Part print with two shaded views. Sizes in mm from the minimum x, y, z corner. Give positions to 0.01 mm unless a question says otherwise; leave off trailing zeros. Write each loop counter-clockwise with the first axis right and the second up, starting at its lowest first coordinate (ties: lowest second). Pieces come first, ordered by that corner, then holes.
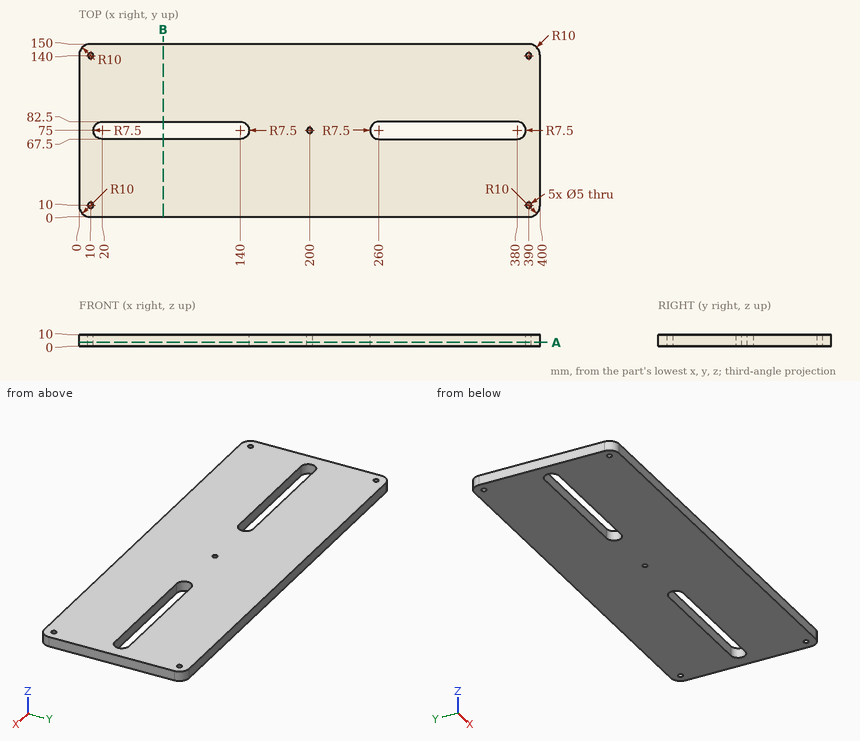
1) Saw through at A-A (z = 3.5). Write the cut outline in (x, y), and give its area (3 significant figures).
Check result:
outline: (0, 10) arc R10 ccw to (10, 0) - (390, 0) arc R10 ccw to (400, 10) - (400, 140) arc R10 ccw to (390, 150) - (10, 150) arc R10 ccw to (0, 140) - close; hole circle Ø5 at (10, 10); hole circle Ø5 at (10, 140); hole (20, 67.5) - (140, 67.5) arc R7.5 ccw to (140, 82.5) - (20, 82.5) arc R7.5 ccw to start; hole circle Ø5 at (200, 75); hole (260, 67.5) - (380, 67.5) arc R7.5 ccw to (380, 82.5) - (260, 82.5) arc R7.5 ccw to start; hole circle Ø5 at (390, 10); hole circle Ø5 at (390, 140)
area: 55,900 mm2
2) Drill centre lines: L1, parallel to X at y = 140, z = 3; L2, parallel to Y at x = 390, z = 3.75; L3, parallel to Y at x = 73, z = 2.25. Where is each one in solid material? Low to high.
Check result:
L1: x = 0 to 7.5, 12.5 to 387.5, 392.5 to 400
L2: y = 0 to 7.5, 12.5 to 137.5, 142.5 to 150
L3: y = 0 to 67.5, 82.5 to 150
3) Saw through at B-B (x = 73). Write the cut outline in (y, z).
Check result:
outline: (0, 0) - (67.5, 0) - (67.5, 10) - (0, 10) - close; (82.5, 0) - (150, 0) - (150, 10) - (82.5, 10) - close
